Part model, mm, in its own coordinate system. Face numbers are marked on the shaded views. A direction names the side the tool comes from. Round coordinates to 2 decimals unless told otherwise and drop trailing zeros. Loops run counter-clockwise (first coordinate to the right, second up) from the corner with the lowest first, then second, coordinate; pieces in that order, holes last. Notation, with made-up numbers: M 73.25,-4.5 L 123.25,-4.5 A29 cw 123.25,18.5 Z; hole C 73.25,77.25 d9. An arc over 180 degrees is marked long. Answer as CSV lines item,"result". Start each with the question number.
Item 1: Band-saw the part on A-A (y = -43.5). Give the cut face in (x, z), and give its area (4 significant figures).
Item 2: Band-saw the part on C-C (y = -5.25). Give the cut face in (x, z), and give its area (4 significant figures).
Item 3: Which spindle directions (+Z, -Z, +X, -X, +Y, -Y) get a long thin tool onto all of the face, cutting with end or side? Do the marked faces 1, 2, 3 and 4. Say none if no direction does.
Item 4: Band-saw the part on D-D (z = 33.5). Give the cut face in (x, y), and give its area (3 significant figures).
Item 5: Wall check: line 1 (X direction, y = -5, z = 6); line 2 (Y direction, x = 5, z = 6); line 3 (Y direction, x = 25, z = 7). Give the ranges that are in metal, low to high.
Item 6: Band-saw the part on B-B (z = 5.5). Give the cut face in (x, y).
Item 7: Drop flat-ended pins along their axis: pin 1 Ø10 at (x, y) = (45, -8.5) entering from +Z; pin 2 Ø6.5 at (y, z) = (-26, 49) entering from -X; pin 3 Ø2 at (x, z) = (41.5, 33) entering from +Y; pin 4 Ø5 at (x, y) = (26, -24.5) entering from +Z. Give the stop position or say it passes through.
Item 8: Mould opens along X. For the marked faces 5, 6 and 7 say: pulls with the +X half, pulls with the -X half, needs draft (parallel to the pull), parting line crosses it, or undercut.
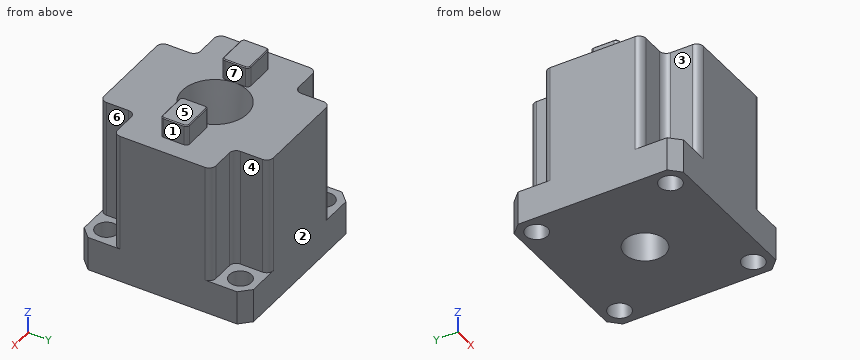
```python
from build123d import *

# Parameters (mm, degrees)
SKETCH_1_W          = 50
SKETCH_1_H          = 50
EXTRUDE_1_DEPTH     = 45
SKETCH_4_W          = 10.5
SKETCH_4_H          = 10.5
CUT_EXTRUDE_1_DEPTH = 35
FILLET_1_R          = 2
CHAMFER_1_SIZE      = 3
SKETCH_5_R          = 3.25
CUT_EXTRUDE_2_DEPTH = 11
SKETCH_7_W          = 10
SKETCH_7_H          = 8
EXTRUDE_4_DEPTH     = 6
FILLET_2_R          = 1
CHAMFER_2_SIZE      = 0.25


with BuildPart() as part:
    # 草图1 → 凸台-拉伸1 (new body)
    with BuildSketch(Plane.XY):
        with Locations((25, -25)):
            Rectangle(SKETCH_1_W, SKETCH_1_H)
    extrude(amount=EXTRUDE_1_DEPTH)

    # 草图4 → 切除-拉伸1 (cut)
    with BuildSketch(Plane.XY.offset(45)):
        with Locations((5.25, -5.25)):
            Rectangle(SKETCH_4_W, SKETCH_4_H)
        with Locations((44.75, -5.25)):
            Rectangle(SKETCH_4_W, SKETCH_4_H)
        with Locations((44.75, -44.75)):
            Rectangle(SKETCH_4_W, SKETCH_4_H)
        with Locations((5.25, -44.75)):
            Rectangle(SKETCH_4_W, SKETCH_4_H)
    extrude(amount=-CUT_EXTRUDE_1_DEPTH, mode=Mode.SUBTRACT)

    # 圆角1
    fillet_1_edges = [part.edges().sort_by_distance(p)[0] for p in [
        (0, -39.5, 27.5),
        (10.5, -39.5, 27.5),
        (10.5, -50, 27.5),
        (39.5, -50, 27.5),
        (39.5, -39.5, 27.5),
        (50, -39.5, 27.5),
        (50, -10.5, 27.5),
        (39.5, -10.5, 27.5),
        (39.5, 0, 27.5),
        (0, -10.5, 27.5),
        (10.5, 0, 27.5),
        (10.5, -10.5, 27.5),
    ]]
    fillet(fillet_1_edges, radius=FILLET_1_R)

    # 倒角1
    chamfer_1_edges = [part.edges().sort_by_distance(p)[0] for p in [
        (0, 0, 5),
        (50, 0, 5),
        (50, -50, 5),
        (0, -50, 5),
    ]]
    chamfer(chamfer_1_edges, length=CHAMFER_1_SIZE)

    # 草图5 → 切除-拉伸2 (cut, through all)
    with BuildSketch(Plane.XY.offset(10)):
        with Locations((5.25, -5.25)):
            Circle(SKETCH_5_R)
        with Locations((44.75, -5.25)):
            Circle(SKETCH_5_R)
        with Locations((44.75, -44.75)):
            Circle(SKETCH_5_R)
        with Locations((5.25, -44.75)):
            Circle(SKETCH_5_R)
    extrude(amount=-CUT_EXTRUDE_2_DEPTH, mode=Mode.SUBTRACT)

    # 草图6 → 切除-旋转1 (revolve, cut)
    with BuildSketch(Plane(origin=(25, 0, 0), x_dir=(0, 0, -1), z_dir=(1, 0, 0))):
        Polygon((-45, -15.4), (-45, -25), (0, -25), (0, -19), (-20.314285805, -19), align=None)
    revolve(axis=Axis((25, -25, 0), (0, 0, 1)), mode=Mode.SUBTRACT)

    # 草图7 → 凸台-拉伸4 (add)
    with BuildSketch(Plane.XY.offset(45)):
        with Locations((39.6, -25)):
            Rectangle(SKETCH_7_W, SKETCH_7_H)
        with Locations((10.4, -25)):
            Rectangle(SKETCH_7_W, SKETCH_7_H)
    extrude(amount=EXTRUDE_4_DEPTH)

    # 圆角2
    fillet_2_edges = [part.edges().sort_by_distance(p)[0] for p in [
        (34.6, -21, 48),
        (34.6, -29, 48),
        (44.6, -29, 48),
        (44.6, -21, 48),
        (15.4, -29, 48),
        (15.4, -21, 48),
        (5.4, -21, 48),
        (5.4, -29, 48),
    ]]
    fillet(fillet_2_edges, radius=FILLET_2_R)

    # 倒角2
    chamfer_2_edges = [part.edges().sort_by_distance(p)[0] for p in [
        (5.4, -25, 51),
        (10.4, -21, 51),
        (15.4, -25, 51),
        (10.4, -29, 51),
        (15.107106781, -21.292893219, 51),
        (15.107106781, -28.707106781, 51),
        (5.692893219, -28.707106781, 51),
        (5.692893219, -21.292893219, 51),
        (34.6, -25, 51),
        (39.6, -21, 51),
        (39.6, -29, 51),
        (44.6, -25, 51),
        (44.307106781, -28.707106781, 51),
        (34.892893219, -28.707106781, 51),
        (44.307106781, -21.292893219, 51),
        (34.892893219, -21.292893219, 51),
    ]]
    chamfer(chamfer_2_edges, length=CHAMFER_2_SIZE)


solid = part.part
```
Answer block:
1,outline,"M 0,0 L 2.25,0 L 2.25,10 L 0,10 Z; M 8.25,0 L 41.75,0 L 41.75,10 L 39.5,10 L 39.5,45 L 10.5,45 L 10.5,10 L 8.25,10 Z; M 47.75,0 L 50,0 L 50,10 L 47.75,10 Z"
1,area,"1,395 mm^2"
2,outline,"M 0,0 L 2,0 L 2,10 L 0,10 Z; M 8.5,0 L 41.5,0 L 41.5,10 L 39.5,10 L 39.5,45 L 10.5,45 L 10.5,10 L 8.5,10 Z; M 48,0 L 50,0 L 50,10 L 48,10 Z"
2,area,"1,385 mm^2"
3,face 1,"+Z, +X, +Y, -Y"
3,face 2,"+Z, -Z, +X, -X, +Y"
3,face 3,"+Z, -X, -Y"
3,face 4,"+Z, +X, +Y"
4,outline,"M 0,-37.5 A2 ccw 2,-39.5 L 8.5,-39.5 A2 cw 10.5,-41.5 L 10.5,-48 A2 ccw 12.5,-50 L 37.5,-50 A2 ccw 39.5,-48 L 39.5,-41.5 A2 cw 41.5,-39.5 L 48,-39.5 A2 ccw 50,-37.5 L 50,-12.5 A2 ccw 48,-10.5 L 41.5,-10.5 A2 cw 39.5,-8.5 L 39.5,-2 A2 ccw 37.5,0 L 12.5,0 A2 ccw 10.5,-2 L 10.5,-8.5 A2 cw 8.5,-10.5 L 2,-10.5 A2 ccw 0,-12.5 Z; hole C 25,-25 d15.85"
4,area,"1,860 mm^2"
5,line 1,"x = 0 to 2.01, 8.49 to 41.51, 47.99 to 50"
5,line 2,"y = -50 to -47.99, -41.51 to -8.49, -2.01 to 0"
5,line 3,"y = -50 to -31, -19 to 0"
6,outline,"M 0,-47 L 3,-50 L 47,-50 L 50,-47 L 50,-3 L 47,0 L 3,0 L 0,-3 Z; hole C 5.25,-44.75 d6.5; hole C 5.25,-5.25 d6.5; hole C 25,-25 d12; hole C 44.75,-44.75 d6.5; hole C 44.75,-5.25 d6.5"
7,pin 1,"stops at z = 45"
7,pin 2,"stops at x = 5.4"
7,pin 3,"stops at y = -10.23"
7,pin 4,"passes through"
8,face 5,"needs draft"
8,face 6,"pulls with the +X half"
8,face 7,"undercut"
